Autodesk Inventor part; units mm, degrees
ref_plane "YZ Plane" through (0, 0, 0) normal (1, 0, 0) x (0, 1, 0)
ref_plane "XZ Plane" through (0, 0, 0) normal (0, 1, 0) x (-1, 0, 0)
ref_plane "XY Plane" through (0, 0, 0) normal (0, 0, 1) x (1, 0, 0)
sketch "Sketch1" plane through (0, 0, 0) normal (0, 1, 0) x (-1, 0, 0)
  line L0 (-33.5, -50) -> (33.5, -50)
  line L1 (33.5, -50) -> (33.5, 50)
  line L2 (33.5, 50) -> (-33.5, 50)
  line L3 (-33.5, 50) -> (-33.5, -50)
  line L4 (-33.5, -50) -> (33.5, 50) construction
  line L5 (33.5, -50) -> (-33.5, 50) construction
  point P0 (0, 0)
  dimension "d0" = 67
  dimension "d1" = 100
extrude "Extrusion1" add sketch "Sketch1" along normal blind 2.8
sketch "Sketch2" plane through (0, 2.8, 0) normal (0, 1, 0) x (1, 0, 0)
  line L0 (33.5, 50) -> (-33.5, 50)
  line L1 (-32.5, -22) -> (23.5, -22)
  line L2 (23.5, -22) -> (23.5, 48)
  line L3 (23.5, 48) -> (-32.5, 48)
  line L4 (-32.5, 48) -> (-32.5, -22)
  line L5 (-32.5, -22) -> (23.5, 48) construction
  line L6 (23.5, -22) -> (-32.5, 48) construction
  line L7 (-33.5, 50) -> (-33.5, -50)
  point P0 (0, 0)
  point P1 (-4.5, 13)
  point P2 (-4.5, 13)
  dimension "d5" = 56
  dimension "d6" = 70
  dimension "d7" = 2
  dimension "d22" = 1
extrude "Extrusion2" cut sketch "Sketch2" against normal blind 1.7
sketch "Sketch3" plane through (0, 1.1, 0) normal (0, 1, 0) x (1, 0, 0)
  line L0 (23.5, -22) -> (-32.5, -22)
  line L1 (23.5, 48) -> (23.5, -22)
  line L2 (-32.5, 48) -> (23.5, 48)
  line L3 (-32.5, -22) -> (-32.5, 48)
  line L4 (-30.5, 46) -> (19.5, 46)
  line L5 (19.5, 46) -> (19.5, -20)
  line L6 (19.5, -20) -> (-30.5, -20)
  line L7 (-30.5, -20) -> (-30.5, 46)
  point P0 (0, 0)
  dimension "d10" = 2
  dimension "d11" = 2
  dimension "d12" = 4
  dimension "d13" = 2
extrude "Extrusion3" cut sketch "Sketch3" against normal blind 0.4 contours L4 L5 L6 L7
sketch "Sketch8" plane through (0, 0.7, 0) normal (0, 1, 0) x (1, 0, 0)
  line L0 (-30.5, 46) -> (19.5, 46)
  line L1 (-33.5, 50) -> (-33.5, -50)
  line L2 (33.5, 50) -> (-33.5, 50)
  line L3 (14.5, -6.5) -> (-23.5, -6.5)
  line L4 (-23.5, -6.5) -> (-23.5, 46)
  line L5 (-23.5, 46) -> (14.5, 46)
  line L6 (14.5, 46) -> (14.5, -6.5)
  point P0 (0, 0)
  dimension "d36" = 10
  dimension "d37" = 4
  dimension "d38" = 38
  dimension "d39" = 52.5
extrude "Extrusion7" cut sketch "Sketch8" against normal up to next
sketch "Sketch4" plane through (0, 2.8, 0) normal (0, 1, 0) x (1, 0, 0)
  line L0 (23.5, 48) -> (23.5, -22)
  line L1 (33.5, -50) -> (33.5, 50)
  line L2 (23.5, 44) -> (32.5, 44)
  line L3 (32.5, 44) -> (32.5, 29)
  line L4 (32.5, 29) -> (23.5, 29)
  line L5 (23.5, 29) -> (23.5, 44)
  line L6 (-32.5, 48) -> (23.5, 48)
  point P0 (0, 0)
  dimension "d18" = 1
  dimension "d21" = 15
  dimension "d33" = 4
extrude "Extrusion4" cut sketch "Sketch4" against normal up to surface (1.7 mm away)
sketch "Sketch6" plane through (33.5, 0, 50) normal (1, 0, 0) x (0, 0, -1)
  line L0 (100, 0) -> (100, 2.8)
  line L1 (0, 2.8) -> (100, 2.8)
  line L2 (0, 0) -> (0, 2.8)
  line L3 (3, 2.8) -> (8, 2.8)
  line L4 (8, 2.8) -> (8, 1.6)
  line L5 (8, 1.6) -> (3, 1.6)
  line L6 (3, 1.6) -> (3, 2.8)
  line L7 (92, 2.8) -> (97, 2.8)
  line L8 (97, 2.8) -> (97, 1.6)
  line L9 (97, 1.6) -> (92, 1.6)
  line L10 (92, 1.6) -> (92, 2.8)
  point P0 (50, 0)
  dimension "d23" = 5
  dimension "d24" = 1.2
  dimension "d25" = 3
  dimension "d26" = 5
  dimension "d27" = 1.2
  dimension "d28" = 3
extrude "Extrusion5" add sketch "Sketch6" along normal blind 1 draft -10
sketch "Sketch7" plane through (-33.5, 0, -50) normal (-1, 0, 0) x (0, 0, 1)
  line L0 (92, 1.6) -> (97, 1.6)
  line L1 (97, 1.6) -> (97, 2.8)
  line L2 (97, 2.8) -> (92, 2.8)
  line L3 (92, 2.8) -> (92, 1.6)
  line L4 (3, 2.8) -> (3, 1.6)
  line L5 (8, 2.8) -> (3, 2.8)
  line L6 (3, 1.6) -> (8, 1.6)
  line L7 (8, 1.6) -> (8, 2.8)
  point P0 (50, 0)
extrude "Extrusion6" add sketch "Sketch7" along normal blind 1 draft -10
fillet "Fillet1" radius 0.5 4 edges at (-23.5, 0, -19.75) (-4.5, 0, -46) (-4.5, 0, 6.5) (14.5, 0, -19.75)
properties part number "TopTouch"
Input: part model. Units: mm. Frame: model coordinates. A direction names the side the tool comes from. Give positions to 0.01 mm unless a question says otherwise; leave off trailing zeros. Order: outer loops, then holes, each group sorted by start corner. A loop starts at its lowest first (then second) coordinate and runs counter-clockwise, first axis right, second up.
1. Cut plane D-D (x = 27). Return loops of the section in (y, z).
Computed:
outline: (0, -50) - (2.8, -50) - (2.8, -44) - (1.1, -44) - (1.1, -29) - (2.8, -29) - (2.8, 50) - (0, 50) - close
2. Pin query (flat end, axial travel): pin 1 Ø0.5 at (y, z) = (2, -38) entering from -X; pin 2 Ø5 at (x, z) = (21, 2.5) entering from -Y. Return the tip coordinate at first contact, or that it passes through.
Computed:
pin 1: stops at x = -33.5
pin 2: stops at y = 0
3. Cut plane B-B (x = -11). Return loops of the section in (y, z), and give its area (3 significant figures).
Computed:
outline: (0, -50) - (2.8, -50) - (2.8, -48) - (1.1, -48) - (1.1, -46) - (0.5, -46) arc R0.5 ccw to (0, -46.5) - close; (0, 7) arc R0.5 ccw to (0.5, 6.5) - (0.7, 6.5) - (0.7, 20) - (1.1, 20) - (1.1, 22) - (2.8, 22) - (2.8, 50) - (0, 50) - close
area: 97.7 mm2
4. Draft query along X for faces 3 (the face through (-6, 0.7, 9)), 4 (the face through (-33.5, 1, -1)), 5 (the face through (8, 2.8, 34)), 6 (the face through (22, 1.1, -16)). Return one class per face: released by +X, released by -X, zero draft, split by the parting line, or undercut.
Computed:
face 3: undercut
face 4: released by -X
face 5: zero draft
face 6: undercut
5. Cut plane C-C (z = -39). Return loops of the section in (x, y).
Computed:
outline: (-33.5, 0) - (-24, 0) arc R0.5 ccw to (-23.5, 0.5) - (-23.5, 0.7) - (-30.5, 0.7) - (-30.5, 1.1) - (-32.5, 1.1) - (-32.5, 2.8) - (-33.5, 2.8) - close; (14.5, 0.5) arc R0.5 ccw to (15, 0) - (33.5, 0) - (33.5, 2.8) - (32.5, 2.8) - (32.5, 1.1) - (19.5, 1.1) - (19.5, 0.7) - (14.5, 0.7) - close
6. Cut plane A-A (z = 0.5). Return loops of the section in (x, y).
Computed:
outline: (-33.5, 0) - (-24, 0) arc R0.5 ccw to (-23.5, 0.5) - (-23.5, 0.7) - (-30.5, 0.7) - (-30.5, 1.1) - (-32.5, 1.1) - (-32.5, 2.8) - (-33.5, 2.8) - close; (14.5, 0.5) arc R0.5 ccw to (15, 0) - (33.5, 0) - (33.5, 2.8) - (23.5, 2.8) - (23.5, 1.1) - (19.5, 1.1) - (19.5, 0.7) - (14.5, 0.7) - close
7. Line query: probe 1 along Z at (x, y) = (-24, 0.85); probe 2 along Z at (x, y) = (-24, 1.55); probe 3 along X at (y, z) = (1.4, 11). Output: solid intervals per line, ascending.
Computed:
probe 1: z = -50 to -46, 20 to 50
probe 2: z = -50 to -48, 22 to 50
probe 3: x = -33.5 to -32.5, 23.5 to 33.5
8. Set-up query: faces 1 (the face through (33.5, 1, 1)), 2 (the face through (0, 1, 50)). Return all of +Z, -Z, +X, -X, +Y, -Y with unobstructed straight access to the full face (end or side cutting, diameter ignored); none if empty.
Computed:
face 1: +X, -Y
face 2: +Z, +X, -X, +Y, -Y
